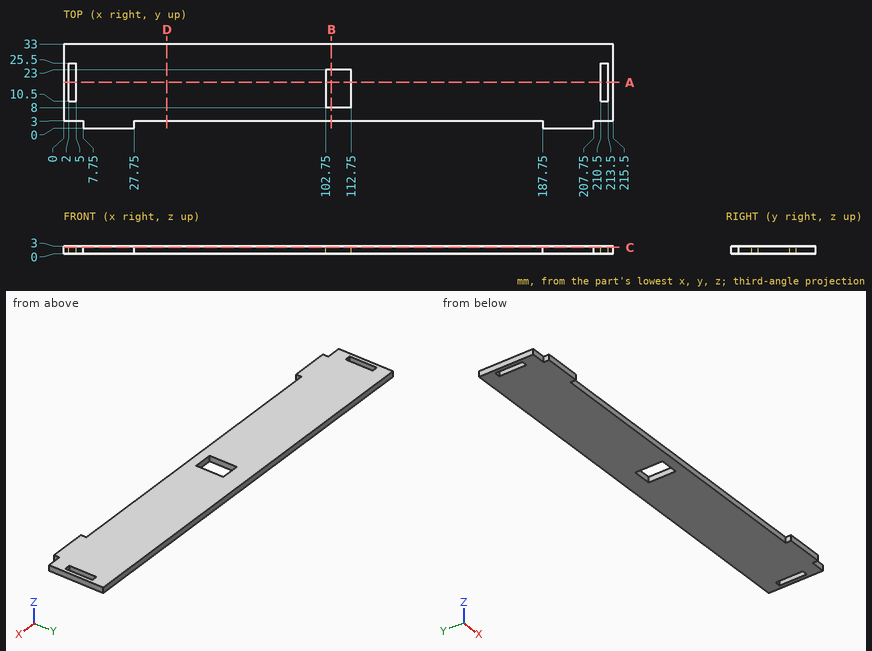
Can you work these out from the drawing? Everything is in mm from the part's minimum corner. Coordinates: 2 decimals unless noted, no trailing zeros. Loops run counter-clockwise (first coordinate to the right, second up) from the corner with the lowest first, then second, coordinate; pieces in that order, holes last. Notation, with made-up numbers: M 1,61 L 41,61 A31 ccw 41,98 Z; hole C -5,88 d6. An arc over 180 degrees is marked long. Put each result on its own line as item: value. Start each with the question number.
(1) Suppose I cut it at D-D on x = 40.5. Please give me the cut outline in (y, z), then the cut area to 3 significant figures.
(2) Suppose I cut it at B-B on x = 105. Please give me the cut outline in (y, z), then the cut area to 3 significant figures.
(3) I need wall thicknesses on line 1 (X direction, y = 20, z = 0.95); line 2 (X direction, y = 23.5, z = 2.3); line 3 (Y direction, x = 105.5, z = 2.05). Which ranges of each line are inside material? Lowest first, please. Write a range as from..to.
(4) Will these pins go through, and if not, where does the flat tip stop? P1, Ø0.9, axis at x = 3, z = 1.5, coming from the -Y side; P2, Ø1.5, axis at y = 1.5, z = 1.5, coming from the -X side.
(5) Suppose I cut it at A-A on y = 18. Please give me the cut outline in (x, z), then the cut area to 4 significant figures.
(6) Suppose I cut it at C-C on z = 2.5. Please give me the cut outline in (x, y).
Solutions:
1. outline: M 3,0 L 33,0 L 33,3 L 3,3 Z
1. area: 90.0 mm2
2. outline: M 3,0 L 8,0 L 8,3 L 3,3 Z; M 23,0 L 33,0 L 33,3 L 23,3 Z
2. area: 45.0 mm2
3. line 1: x = 0..2, 5..102.75, 112.75..210.5, 213.5..215.5
3. line 2: x = 0..2, 5..210.5, 213.5..215.5
3. line 3: y = 3..8, 23..33
4. P1: stops at y = 3
4. P2: stops at x = 7.75
5. outline: M 0,0 L 2,0 L 2,3 L 0,3 Z; M 5,0 L 102.75,0 L 102.75,3 L 5,3 Z; M 112.75,0 L 210.5,0 L 210.5,3 L 112.75,3 Z; M 213.5,0 L 215.5,0 L 215.5,3 L 213.5,3 Z
5. area: 598.5 mm2
6. outline: M 0,3 L 7.75,3 L 7.75,0 L 27.75,0 L 27.75,3 L 187.75,3 L 187.75,0 L 207.75,0 L 207.75,3 L 215.5,3 L 215.5,33 L 0,33 Z; hole M 2,10.5 L 5,10.5 L 5,25.5 L 2,25.5 Z; hole M 102.75,8 L 112.75,8 L 112.75,23 L 102.75,23 Z; hole M 210.5,10.5 L 213.5,10.5 L 213.5,25.5 L 210.5,25.5 Z
